Model file for the job. Use its own axes, mm. Face numbers are marked on the shaded views. Coordinates: 2 decimals unless noted, no trailing zeros. Write each loop counter-clockwise with the first axis right and the second up, starting at its lowest first coordinate (ties: lowest second). Pieces come first, ordered by that corner, then holes. Notation, with made-up numbers: (69, -31) - (77, -31) arc R9 cw to (77, -25) - close; hole circle Ø7 at (-21, 35). An arc over 180 degrees is marked (long way). Put each result on its own line as item: value. Start each with the question number.
1. Saw through at A-A, the plane y = 0. Write the cut outline in (x, z).
2. Saw through at B-B, the plane z = 1. Write the cut outline in (x, y), plus the area to 3 significant figures.
3. Saw through at D-D, the plane z = 5.5. Write the cut outline in (x, y), plus the area to 3 significant figures.
4. Drop flat-ended pins along their axis: P1, Ø1, axis at x = -1.5, z = -0.5, coming from the -Y side; P2, Ø1.5, axis at y = 18, z = 8, coming from the -X side; P3, Ø1, axis at x = 6.5, z = -0.5, coming from the -Y side. Give the stop position or say it passes through.
5. Pull direction X, two halves, no side cores. Call the marked faces 1, 2 and 3: released by +X, released by -X, zero draft, split by the parting line, or undercut.
6. Drill centre lines: L1, parallel to Y at x = 0, z = 1.5; L2, parallel to Y at x = 0, z = 5.5; L3, parallel to Z at x = 22, y = -18. Where is each one in solid material? Low to high. Write a range as from..to.
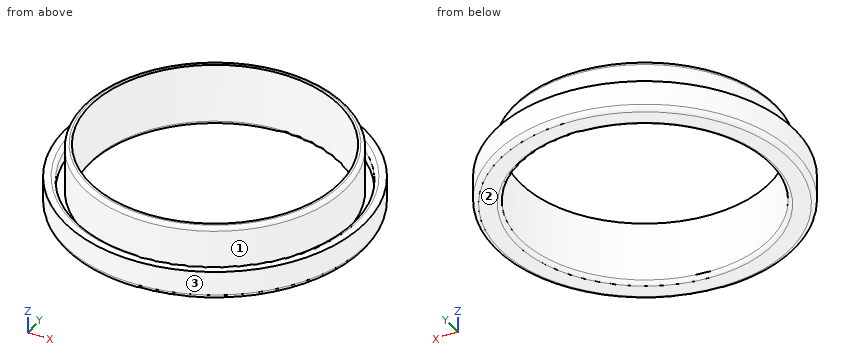
```python
from build123d import *

# Parameters (mm, degrees)
F0_R     = 31
F0_R_2   = 28.75
F0_R_3   = 27.1
F0_R_4   = 25.8
F1_DEPTH = 3
F2_DEPTH = 10
F3_DEPTH = 3
F4_DEPTH = 25
F5_R     = 0.8
F6_R     = 1


with BuildPart() as f1:
    # F0 (on Top) → F1 (new body)
    with BuildSketch(Plane.XY):
        Circle(F0_R)
        Circle(F0_R_2, mode=Mode.SUBTRACT)
        Circle(F0_R_2)
        Circle(F0_R_3, mode=Mode.SUBTRACT)
        Circle(F0_R_3)
        Circle(F0_R_4, mode=Mode.SUBTRACT)
    extrude(amount=-F1_DEPTH)

    # F0 (on Top) → F2 (join)
    with BuildSketch(Plane.XY):
        Circle(F0_R_3)
        Circle(F0_R_4, mode=Mode.SUBTRACT)
    extrude(amount=F2_DEPTH)

    # F0 (on Top) → F3 (join)
    with BuildSketch(Plane.XY):
        Circle(F0_R)
        Circle(F0_R_2, mode=Mode.SUBTRACT)
    extrude(amount=F3_DEPTH)

    # F0 (on Top) → F4 (cut)
    with BuildSketch(Plane.XY):
        Circle(F0_R_4)
    extrude(amount=F4_DEPTH, mode=Mode.SUBTRACT)

    # F5
    f5_edges = [f1.edges().sort_by_distance(p)[0] for p in [
        (-25.8, 0, -3),
        (-28.75, 0, 3),
        (-27.1, 0, 10),
    ]]
    fillet(f5_edges, radius=F5_R)

    # F6
    f6_edges = [f1.edges().sort_by_distance(p)[0] for p in [
        (-31, 0, -3),
    ]]
    fillet(f6_edges, radius=F6_R)


solid = f1.part
```
Final values:
1. outline: (-31, -2) arc R1 ccw to (-30, -3) - (-26.6, -3) arc R0.8 ccw to (-25.8, -2.2) - (-25.8, 10) - (-26.3, 10) arc R0.8 ccw to (-27.1, 9.2) - (-27.1, 0) - (-28.75, 0) - (-28.75, 2.2) arc R0.8 ccw to (-29.55, 3) - (-31, 3) - close; (25.8, -2.2) arc R0.8 ccw to (26.6, -3) - (30, -3) arc R1 ccw to (31, -2) - (31, 3) - (29.55, 3) arc R0.8 ccw to (28.75, 2.2) - (28.75, 0) - (27.1, 0) - (27.1, 9.2) arc R0.8 ccw to (26.3, 10) - (25.8, 10) - close
2. outline: circle Ø62 at (0, 0); circle Ø54.2 at (0, 0); hole circle Ø57.5 at (0, 0); hole circle Ø51.6 at (0, 0)
2. area: 638 mm²
3. outline: circle Ø54.2 at (0, 0); hole circle Ø51.6 at (0, 0)
3. area: 216 mm²
4. P1: stops at y = -30.98
4. P2: stops at x = -20.9
4. P3: stops at y = -30.41
5. face 1: undercut
5. face 2: zero draft
5. face 3: split by the parting line
6. L1: y = -31..-28.75, -27.1..-25.8, 25.8..27.1, 28.75..31
6. L2: y = -27.1..-25.8, 25.8..27.1
6. L3: z = -3..0
